Model file for the job. Use its own axes, mm. A direction names the side the tool comes from. Round coordinates to 2 decimals unless told otherwise and drop trailing zeros. Order: outer loops, then holes, each group sorted by start corner. A loop starts at its lowest first (then second) coordinate and runs counter-clockwise, first axis right, second up. Notation, with made-up numbers: M 4,-9 L 23,-9 A30 cw 23,24 Z; hole C -20.5,-23.5 d11. An arc over 180 degrees is marked long. Return JSON: item names as keys, results as strings. Group by question number.
Item 1: Pin check, flat tips, straight feed: pin 1 Ø12 at (x, y) = (-6, 9) entering from -Z; pin 2 Ø1 at (x, y) = (7, 5.5) entering from -Z; pin 3 Ø8 at (y, z) = (13.5, -8) entering from +X; pin 4 Ø1 at (x, y) = (1, 11) entering from +Z. Stop position of each tip, or through.
Item 2: Slice it at D-D on y = 11.25. Write the cut outline in (x, z).
Item 3: Slice it at C-C on y = 18.25. Write the cut outline in (x, z), then the cut area to 3 significant figures.
Item 4: Which spindle directions (+Z, -Z, +X, -X, +Y, -Y) get a long thin tool onto all of the face, cutting with end or side? Do faces 1 (the face through (5, 17, -2)), 2 (the face through (0, 22, 0)). Say none if no direction does.
Item 5: Probe line 1 along Y through (x, z) = (-4, 8.25); line 2 along Z through (x, y) = (-0.25, 4.25); line 3 along Z through (x, y) = (-8, 18.25). List the from-to ranges inside material, lowest first.
Item 6: Slice it at B-B on z = 0. Write the cut outline in (x, y), then the cut area to 3 significant figures.
Item 7: Slice it at A-A on x = 0. Write the cut outline in (y, z), then the cut area to 3 significant figures.
Solid Edge part; units mm, degrees
sketch "Sketch1" plane through (0, 0, 0) normal (0, -1, 0) x (1, 0, 0)
  circle A0 centre (0, 0) radius 5.15
extrude "Protrusion1" add sketch "Sketch1" against normal blind 17
chamfer "Fase_1" distance 1 angle 45 1 edges at (-5.15, 0, 0)
sketch "Sketch2" plane through (0, 17, 0) normal (0, 1, 0) x (-1, 0, 0)
  circle A0 centre (0, 0) radius 10
extrude "Extrusionsausprägung_2" add sketch "Sketch2" along normal blind 5
Output values:
{
 "1": {"pin 1": "z = -5.15", "pin 2": "through", "pin 3": "x = 7.95", "pin 4": "z = 5.13"},
 "2": {"outline": "C 0,0 d10.3"},
 "3": {"outline": "C 0,0 d20", "area": "314 mm²"},
 "4": {"face 1": "-Y", "face 2": "+Z, -Z, +X, -X, +Y"},
 "5": {"line 1": "17 to 22", "line 2": "-5.14 to 5.14", "line 3": "-6 to 6"},
 "6": {"outline": "M -10,17 L -5.15,17 L -5.15,1 L -4.15,0 L 4.15,0 L 5.15,1 L 5.15,17 L 10,17 L 10,22 L -10,22 Z", "area": "274 mm²"},
 "7": {"outline": "M 0,-4.15 L 1,-5.15 L 17,-5.15 L 17,-10 L 22,-10 L 22,10 L 17,10 L 17,5.15 L 1,5.15 L 0,4.15 Z", "area": "274 mm²"}
}
